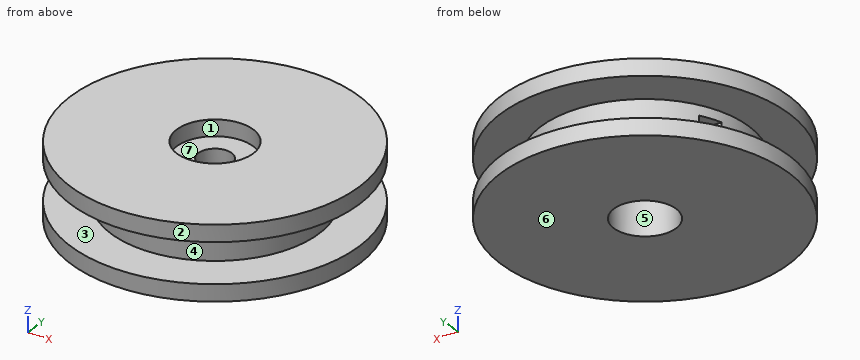
```python
from build123d import *

# Parameters (mm, degrees)
CROQUIS1_R                 = 10.75
SALIENTE_EXTRUIR1_DEPTH    = 5.5
CROQUIS3_R                 = 2.85
CORTAR_EXTRUIR1_DEPTH      = 1.2
CROQUIS4_R                 = 1.25
CORTAR_EXTRUIR2_DEPTH      = 17.167096214
CROQUIS5_R                 = 2.32
CORTAR_EXTRUIR3_DEPTH      = 2.7
CORTAR_EXTRUIR4_DEPTH      = 17.167096214
CORTAR_EXTRUIR4_DEPTH_BACK = 17.167096214
CROQUIS6_W                 = 1.5
CROQUIS6_H                 = 1.5


with BuildPart() as part:
    # Croquis1 → Saliente-Extruir1 (new body)
    with BuildSketch(Plane.XY):
        Circle(CROQUIS1_R)
    extrude(amount=SALIENTE_EXTRUIR1_DEPTH)

    # Croquis2 → Cortar-Revolución1 (revolve, cut)
    with BuildSketch(Plane(origin=(0, 0, 0), x_dir=(0, 0, -1), z_dir=(1, 0, 0)), mode=Mode.PRIVATE) as cortar_revoluci_n1_sk:
        Polygon((-5.5, 10.75), (-4.25, 10.75), (-4.25, 7.75), (-1.25, 7.75), (-1.25, 10.75), (0, 10.75), (0, 13.530555933), (-5.5, 13.530555933), align=None)
    revolve(cortar_revoluci_n1_sk.sketch.rotate(Axis((0, 0, 0), (0, 0, 1)), 90), axis=Axis((0, 0, 0), (0, 0, 1)), mode=Mode.SUBTRACT)

    # Croquis3 → Cortar-Extruir1 (cut)
    with BuildSketch(Plane.XY.offset(5.5)):
        Circle(CROQUIS3_R)
    extrude(amount=-CORTAR_EXTRUIR1_DEPTH, mode=Mode.SUBTRACT)

    # Croquis4 → Cortar-Extruir2 (cut, through all)
    with BuildSketch(Plane.XY.offset(5.5)):
        Circle(CROQUIS4_R)
    extrude(amount=-CORTAR_EXTRUIR2_DEPTH, mode=Mode.SUBTRACT)

    # Croquis5 → Cortar-Extruir3 (cut)
    with BuildSketch(Plane(origin=(0, 0, 0), x_dir=(-1, 0, 0), z_dir=(0, 0, -1))):
        Circle(CROQUIS5_R)
    extrude(amount=-CORTAR_EXTRUIR3_DEPTH, mode=Mode.SUBTRACT)

    # Croquis6 → Cortar-Extruir4 (cut, two sides: drawn at the far end of the back side and taken through both)
    with BuildSketch(Plane(origin=(0, 0, 0), x_dir=(0, 0, -1), z_dir=(1, 0, 0)).offset(-CORTAR_EXTRUIR4_DEPTH_BACK)):
        with Locations((-2.75, 3.25)):
            Rectangle(CROQUIS6_W, CROQUIS6_H)
    extrude(amount=CORTAR_EXTRUIR4_DEPTH + CORTAR_EXTRUIR4_DEPTH_BACK, mode=Mode.SUBTRACT)


solid = part.part
```
The listing builds one solid part. Answer for the finished solid, in the listing's coordinates (mm). Face numbers are marked on the shaded views. A direction names the side the tool comes from. Give positions to 0.01 mm unless a question says otherwise; leave off trailing zeros. Loops run counter-clockwise (first coordinate to the right, second up) from the corner with the lowest first, then second, coordinate; pieces in that order, holes last. Notation, with made-up numbers: M 81,0.5 L 99,0.5 A21 cw 99,5.5 Z; hole C 38,-25 d6. An arc over 180 degrees is marked long. One line per item, written item: value.
Q1. Find the intervals of material crossed by line 1 (Y direction, x = 0, z = 2.2); line 2 (Z direction, x = -7.5, y = 3.75); line 3 (Y direction, x = 0, z = 5), in increasing order. Write a range as from..to.
Working result:
line 1: y = -7.75..-2.32, 2.32..2.5, 4..7.75
line 2: z = 0..1.25, 4.25..5.5
line 3: y = -10.75..-2.85, 2.85..10.75
Q2. A cutting plane is placed at C-C on x = -9. Determine the outline of the cut face in (y, z).
Working result:
outline: M -5.88,0 L 5.88,0 L 5.88,1.25 L -5.88,1.25 Z; M -5.88,4.25 L 5.88,4.25 L 5.88,5.5 L -5.88,5.5 Z
Q3. A cutting plane is placed at A-A on x = 0. Determine the outline of the cut face in (y, z).
Working result:
outline: M -10.75,0 L -2.32,0 L -2.32,2.7 L -1.25,2.7 L -1.25,4.3 L -2.85,4.3 L -2.85,5.5 L -10.75,5.5 L -10.75,4.25 L -7.75,4.25 L -7.75,1.25 L -10.75,1.25 Z; M 1.25,2.7 L 2.32,2.7 L 2.32,0 L 10.75,0 L 10.75,1.25 L 7.75,1.25 L 7.75,4.25 L 10.75,4.25 L 10.75,5.5 L 2.85,5.5 L 2.85,4.3 L 1.25,4.3 Z; hole M 2.5,2 L 4,2 L 4,3.5 L 2.5,3.5 Z
Q4. Determine the mould class of the marked faces 4, 5, 6 and 7 for opening direction Y: +Y half, -Y half, draft (parallel to the pull), parting line (faces both ways), or undercut.
Working result:
face 4: parting line
face 5: undercut
face 6: draft
face 7: undercut
Q5. For the marked faces 1, 2 and 3, determine the directions among +Z, -Z, +X, -X, +Y, -Y from which every point of the face is accessible in a straight line to the end or side of a thin tool.
Working result:
face 1: +Z
face 2: +Z, -Z
face 3: none
Q6. Flat-ended cylindrical pins translate along their axes: P1, Ø1, axis at x = 5, z = 3, coming from the +Y side; P2, Ø3, axis at x = 0, y = 1, coming from the +Z side; P3, Ø1.6, axis at x = 1.5, z = 2.5, coming from the -Y side. Find the tip coordinate at first contact, or state that the pin passes through.
Working result:
P1: stops at y = 6.31
P2: stops at z = 4.3
P3: stops at y = -7.72
Q7. A cutting plane is placed at D-D on y = -3.5. Determine the outline of the cut face in (x, z), then the cut area to 3 significant figures.
Working result:
outline: M -10.16,0 L 10.16,0 L 10.16,1.25 L 6.91,1.25 L 6.91,4.25 L 10.16,4.25 L 10.16,5.5 L -10.16,5.5 L -10.16,4.25 L -6.91,4.25 L -6.91,1.25 L -10.16,1.25 Z
area: 92.3 mm^2
Q8. A cutting plane is placed at B-B on y = 0. Determine the outline of the cut face in (x, z).
Working result:
outline: M -10.75,0 L -2.32,0 L -2.32,2.7 L -1.25,2.7 L -1.25,4.3 L -2.85,4.3 L -2.85,5.5 L -10.75,5.5 L -10.75,4.25 L -7.75,4.25 L -7.75,1.25 L -10.75,1.25 Z; M 1.25,2.7 L 2.32,2.7 L 2.32,0 L 10.75,0 L 10.75,1.25 L 7.75,1.25 L 7.75,4.25 L 10.75,4.25 L 10.75,5.5 L 2.85,5.5 L 2.85,4.3 L 1.25,4.3 Z
